Model file for the job. Use its own axes, mm. A direction names the side the tool comes from. Coordinates: 2 decimals unless noted, no trailing zeros. Order: outer loops, then holes, each group sorted by start corner. A loop starts at its lowest first (then second) coordinate and runs counter-clockwise, first axis right, second up. Notation, with made-up numbers: M 88,-9 L 96,-9 A26 cw 96,23 Z; hole C 78.5,62 d3. An arc over 180 degrees is marked long. Return JSON: item names as keys, results as strings.
```python
from build123d import *

# Parameters (mm, degrees)
EXTRUDE_1_DEPTH     = 12
CUT_EXTRUDE_1_DEPTH = 9


with BuildPart() as part:
    # 草图1 → 凸台-拉伸1 (new body)
    with BuildSketch(Plane(origin=(0, 0, 0), x_dir=(1, 0, 0), z_dir=(0, 1, 0))):
        with BuildLine():
            Line((0, 0), (109, 0))
            ThreePointArc((109, 0), (116.778174593, -3.221825407), (120, -11))
            Line((120, -11), (120, -31))
            Line((120, -31), (-11, -31))
            Line((-11, -31), (-11, -11))
            ThreePointArc((-11, -11), (-7.778174593, -3.221825407), (0, 0))
        make_face()
    extrude(amount=EXTRUDE_1_DEPTH)

    # 草图2 → 切除-拉伸1 (cut)
    with BuildSketch(Plane(origin=(0, 12, 0), x_dir=(1, 0, 0), z_dir=(0, 1, 0))):
        with BuildLine():
            Line((-8, -31), (-8, -11))
            ThreePointArc((-8, -11), (-5.656854249, -5.343145751), (0, -3))
            Line((0, -3), (109, -3))
            ThreePointArc((109, -3), (114.656854249, -5.343145751), (117, -11))
            Line((117, -11), (117, -31))
            Line((117, -31), (-8, -31))
        make_face()
    extrude(amount=-CUT_EXTRUDE_1_DEPTH, mode=Mode.SUBTRACT)


solid = part.part
```
Item 1: Drop flat-ended pins along their axis: pin 1 Ø2 at (x, y) = (99, 10) entering from +Z; pin 2 Ø14 at (x, z) = (80, 13.5) entering from +Y; pin 3 Ø3 at (y, z) = (3, 7.5) entering from +X. Give the stop position or say it passes through.
Check result:
{"pin 1": "stops at z = 3", "pin 2": "stops at y = 3", "pin 3": "stops at x = 119.82"}
Item 2: Wall check: line 1 (X direction, y = 4, z = 23.5); line 2 (Y direction, x = 81.5, z = 22). Give the ranges that are in metal, low to high.
Check result:
{"line 1": "x = -11 to -8, 117 to 120", "line 2": "y = 0 to 3"}
Item 3: Saw through at D-D (z = 7). Write the cut outline in (x, y), and give its area (3 significant figures).
Check result:
{"outline": "M -10.25,0 L 119.25,0 L 119.25,12 L 115.93,12 L 115.93,3 L -6.93,3 L -6.93,12 L -10.25,12 Z", "area": "448 mm2"}
Item 4: Saw through at A-A (z = 17.5). Write the cut outline in (x, y), and give its area (3 significant figures).
Check result:
{"outline": "M -11,0 L 120,0 L 120,12 L 117,12 L 117,3 L -8,3 L -8,12 L -11,12 Z", "area": "447 mm2"}
Item 5: Saw through at B-B (y = 4.5). Write the cut outline in (x, z).
Check result:
{"outline": "M -11,11 A11 ccw 0,0 L 109,0 A11 ccw 120,11 L 120,31 L 117,31 L 117,11 A8 cw 109,3 L 0,3 A8 cw -8,11 L -8,31 L -11,31 Z"}
Item 6: Saw through at C-C (x = 22). Write the cut outline in (y, z).
Check result:
{"outline": "M 0,0 L 12,0 L 12,3 L 3,3 L 3,31 L 0,31 Z"}
Item 7: 3-axis set-ups, long thin cutter, end or side, ignore diameter. For faces 4 (the flat face through (120, 6, 21)), 5 (the flat face through (117, 8, 21)): which of +Z, -Z, +X, -X, +Y, -Y reach the whole face in a straight line?
Check result:
{"face 4": "+Z, -Z, +X, +Y, -Y", "face 5": "+Z, +Y"}
Item 8: Pull direction X, two halves, no side cores. Call faces 1 (the flat face through (-11, 6, 21)), 2 (the cylindrical face through (-5.719, 7.563, 5.406)), 3 (the flat face through (54.8, 12, 2.8)): +X half, -X half, draft (parallel to the pull), parting line (faces both ways), or undercut.
Check result:
{"face 1": "-X half", "face 2": "undercut", "face 3": "draft"}
